Work out the finished part from the listing and answer in its coordinate system (mm). Coordinates: 2 decimals unless noted, no trailing zeros. Loops run counter-clockwise (first coordinate to the right, second up) from the corner with the lowest first, then second, coordinate; pieces in that order, holes last. Notation, with made-up numbers: (15.5, 86.25) -> (67.5, 86.25) arc R5 ccw to (67.5, 90.25) -> close; hole circle Ø3 at (26, 70). An arc over 180 degrees is marked (long way). Answer as CSV lines item,"result".
```python
from build123d import *

# Parameters (mm, degrees)
STOCK_LEFT_START                                  = 154.501049255
STOCK_LEFT_CONSOLE_1_OUTLINE_R                    = 2.413
STOCK_LEFT_CONSOLE_1_DEPTH                        = 6.35
SKETCH1_R                                         = 2.413
BOSS_EXTRUDE1_DEPTH                               = 6.35
FILLET1_R                                         = 127
CSK_FOR_8_FLAT_HEAD_MACHINE_SCREW_100_D           = 4.9149
CSK_FOR_8_FLAT_HEAD_MACHINE_SCREW_100_DEPTH       = 36.56137815
CSK_FOR_8_FLAT_HEAD_MACHINE_SCREW_100_CSINK_D     = 8.4328
CSK_FOR_8_FLAT_HEAD_MACHINE_SCREW_100_CSINK_ANGLE = 100


# Read off the part's stored shape, not the designer's step: Stock-Left Console-1
with BuildPart() as part:
    # Stock-Left Console-1 outline → Stock-Left Console-1 (new body)
    with BuildSketch(Plane(origin=(0, 0, 0), x_dir=(0.02679964301193732, 0.9996408236099973, -5.391436833640836e-05), z_dir=(0.999638800759929, -0.0267996972431853, -0.00201103031422956)).offset(STOCK_LEFT_START)):
        Polygon((6894.543157626, 3344.380142713), (5775.416554865, 3260.371330561), (5781.349946418, 3234.680487062), (5961.468932714, 3260.009915697), (6652.879217668, 3311.911600999), (6881.420614343, 3311.911600999), align=None)
        with Locations((5816.052887601, 3253.393618776)):
            Circle(STOCK_LEFT_CONSOLE_1_OUTLINE_R, mode=Mode.SUBTRACT)
        with Locations((5895.828437121, 3259.382082581)):
            Circle(STOCK_LEFT_CONSOLE_1_OUTLINE_R, mode=Mode.SUBTRACT)
        with Locations((5977.356983496, 3265.50213756)):
            Circle(STOCK_LEFT_CONSOLE_1_OUTLINE_R, mode=Mode.SUBTRACT)
        with Locations((6072.652614823, 3272.65563813)):
            Circle(STOCK_LEFT_CONSOLE_1_OUTLINE_R, mode=Mode.SUBTRACT)
        with Locations((6307.675625814, 3290.29797094)):
            Circle(STOCK_LEFT_CONSOLE_1_OUTLINE_R, mode=Mode.SUBTRACT)
        with Locations((6422.028102237, 3298.882000385)):
            Circle(STOCK_LEFT_CONSOLE_1_OUTLINE_R, mode=Mode.SUBTRACT)
        with Locations((6472.834946762, 3302.695887614)):
            Circle(STOCK_LEFT_CONSOLE_1_OUTLINE_R, mode=Mode.SUBTRACT)
        with Locations((6592.955295229, 3311.712890485)):
            Circle(STOCK_LEFT_CONSOLE_1_OUTLINE_R, mode=Mode.SUBTRACT)
        with Locations((6643.762139775, 3315.526777715)):
            Circle(STOCK_LEFT_CONSOLE_1_OUTLINE_R, mode=Mode.SUBTRACT)
        with Locations((6865.316700097, 3322.905070324)):
            Circle(STOCK_LEFT_CONSOLE_1_OUTLINE_R, mode=Mode.SUBTRACT)
    extrude(amount=STOCK_LEFT_CONSOLE_1_DEPTH)

    # Sketch1 → Boss-Extrude1 (add)
    with BuildSketch(Plane(origin=(154.445243594, -4.140581344, -0.310706294), x_dir=(0.002010307996697838, -5.389511255073478e-05, 0.9999979778764931), z_dir=(-0.9996388007599293, 0.026799697243176115, 0.0020110303142280403))):
        Polygon((3259.688501477, 5961.644685781), (3234.3687839, 5781.524334123), (3229.743043385, 5782.592402631), (3254.912621388, 5961.644685781), (3306.77702959, 6653.057767982), (3288.626337955, 6847.775838873), (3290.526309625, 6873.104678319), (3311.540587989, 6881.599164324), (3311.552909679, 6653.057767982), align=None)
        with Locations(Location((3303.484925533, 6857.795366229, 0), (0, 0, 270))):
            Circle(SKETCH1_R, mode=Mode.SUBTRACT)
    extrude(amount=-BOSS_EXTRUDE1_DEPTH)

    # Fillet1
    # the kernel refuses this fillet: 127 mm, written as the material it adds along each edge
    with BuildSketch(Plane(origin=(320.759216191, 5955.187389877, 3254.595333259), x_dir=(-0.026818667254060527, -0.9899007533718392, -0.13920221823153914), z_dir=(0.9996388007599292, -0.026799697243176112, -0.00201103031422804))) as fillet1_piece_1:
        with BuildLine():
            CenterArc((FILLET1_R * 0.0324033639177, FILLET1_R), FILLET1_R, 266.288146769, 3.711853231)
            Line((-FILLET1_R * 0.0323353896511, FILLET1_R * 0.00209775339147), (0, 0))
            Line((0, 0), (FILLET1_R * 0.0324033639177, 0))
        make_face()
    extrude(amount=6.35)
    with BuildSketch(Plane(origin=(339.393178368, 6646.349336581, 3306.459636585), x_dir=(-0.02687504446974266, -0.9968362003292489, -0.07480188298361883), z_dir=(0.9996388007599292, -0.026799697243176112, -0.00201103031422804))) as fillet1_piece_2:
        with BuildLine():
            CenterArc((FILLET1_R * 0.0841067955983, FILLET1_R), FILLET1_R, 260.38470128, 9.61529872)
            Line((-FILLET1_R * 0.0829252189667, FILLET1_R * 0.0140485275074), (0, 0))
            Line((0, 0), (FILLET1_R * 0.0841067955983, 0))
        make_face()
    extrude(amount=6.35)
    # the kernel refuses this fillet: 127 mm, written as the material it takes off along each edge
    with BuildSketch(Plane(origin=(317.880823616, 6841.714103927, 3288.36268402), x_dir=(0.026875044469742655, 0.996836200329251, 0.0748018829835892), z_dir=(0.9996388007599292, -0.026799697243176112, -0.00201103031422804))) as fillet1_2_piece_1:
        with BuildLine():
            CenterArc((FILLET1_R * 0.0841067955983, FILLET1_R), FILLET1_R, 260.38470128, 9.61529872)
            Line((-FILLET1_R * 0.0829252189667, FILLET1_R * 0.0140485275074), (0, 0))
            Line((0, 0), (FILLET1_R * 0.0841067955982, 0))
        make_face()
    extrude(amount=59.757815205, mode=Mode.SUBTRACT)

    # CSK for #8 Flat Head Machine Screw (100)1
    with Locations(Plane(origin=(154.445243594, -4.140581344, -0.310706294), x_dir=(0.002010307996697838, -5.389511255073478e-05, 0.9999979778764931), z_dir=(-0.9996388007599293, 0.026799697243176115, 0.0020110303142280403))):
        with Locations((3322.534925533, 6865.49584281), (3303.484925533, 6857.795366229), (3315.168577933, 6643.940885012), (3311.357429933, 6593.133834917), (3302.346903301, 6473.013000478), (3298.535755302, 6422.205950402), (3289.957891123, 6307.853011342), (3272.328229482, 6072.829049515), (3265.179866736, 5977.533032649), (3259.064207335, 5896.004156434), (3253.080044595, 5816.228284164)):
            CounterSinkHole(CSK_FOR_8_FLAT_HEAD_MACHINE_SCREW_100_D / 2, CSK_FOR_8_FLAT_HEAD_MACHINE_SCREW_100_CSINK_D / 2, depth=CSK_FOR_8_FLAT_HEAD_MACHINE_SCREW_100_DEPTH, counter_sink_angle=CSK_FOR_8_FLAT_HEAD_MACHINE_SCREW_100_CSINK_ANGLE)


solid = part.part
```
(1) A cutting plane is placed at A-A, the plane y = 5837. Write down the section's boundary in (x, z), and give its area (3 significant figures).
Computed values:
outline,"(317.56, 3237.98) -> (323.91, 3237.99) -> (323.96, 3264.83) -> (317.61, 3264.83) -> close"
area,"171 mm2"
(2) A cutting plane is placed at B-B, the plane y = 6082. Write down the section's boundary in (x, z).
Computed values:
outline,"(324.18, 3264.11) -> (330.53, 3264.11) -> (330.57, 3283.21) -> (324.22, 3283.21) -> close"
(3) Consider line 1 along X through (y, z) = (6838, 3332); line 2 along Z through (x, y) = (326.5, 5939); line 3 along X through (y, z) = (6790.5, 3294.5). Determine where each line is inside the solid, lowest interval first.
Computed values:
line 1,"344.58 to 350.93"
line 2,"3252.33 to 3272.48"
line 3,"343.23 to 349.59"
(4) Flat-ended cylindrical pins translate along their axes: pin 1 Ø5 at (y, z) = (6441, 3290) entering from -X; pin 2 Ø1 at (y, z) = (5884.5, 3267.5) entering from -X; pin 3 Ø1 at (y, z) = (6184, 3273.5) entering from +X. Find the tip coordinate at first contact, or state that the pin passes through.
Computed values:
pin 1,"x = 333.79"
pin 2,"x = 318.88"
pin 3,"x = 333.3"
